```python
from build123d import *

# Parameters (mm, degrees)
BOSS_EXTRUDE1_DEPTH  = 19.05
M5_CLEARANCE_HOLE1_D = 5.5
CUT_EXTRUDE1_REACH   = 3.519
SKETCH5_W            = 20.32
SKETCH5_H            = 40.64
CUT_EXTRUDE2_REACH   = 3.519
SKETCH6_R            = 2.032


with BuildPart() as part:
    # Sketch1 → Boss-Extrude1 (new body, symmetric)
    with BuildSketch(Plane(origin=(0, 0, 0), x_dir=(0, 0, -1), z_dir=(1, 0, 0))):
        Polygon((0, 0), (28.380612245, 0), (28.380612245, 63.5), (26.861692245, 63.5), (26.861692245, 1.51892), (0, 1.51892), align=None)
    extrude(amount=BOSS_EXTRUDE1_DEPTH, both=True)

    # M5 Clearance Hole1 (through all)
    with Locations(Plane(origin=(0, 1.51892, 0), x_dir=(1, 0, 0), z_dir=(0, 1, 0))):
        with Locations((-12.7, 13.430846122), (12.7, 13.430846122)):
            Hole(M5_CLEARANCE_HOLE1_D / 2)

    # Sketch5 → Cut-Extrude1 (cut, up to next)
    with BuildSketch(Plane.XY.offset(-26.861692245), mode=Mode.PRIVATE) as cut_extrude1_sk1:
        with Locations((0, 32.50946)):
            Rectangle(SKETCH5_W, SKETCH5_H)
    cut_extrude1_tool1 = extrude(cut_extrude1_sk1.sketch, amount=-CUT_EXTRUDE1_REACH, mode=Mode.PRIVATE) & part.part
    add(cut_extrude1_tool1.solids().sort_by_distance((0, 32.50946, -26.861692))[0], mode=Mode.SUBTRACT)

    # Sketch6 → Cut-Extrude2 (cut, up to next)
    with BuildSketch(Plane.XY.offset(-26.861692245), mode=Mode.PRIVATE) as cut_extrude2_sk1:
        with Locations((-5.969, 57.50946)):
            Circle(SKETCH6_R)
    cut_extrude2_tool1 = extrude(cut_extrude2_sk1.sketch, amount=-CUT_EXTRUDE2_REACH, mode=Mode.PRIVATE) & part.part
    add(cut_extrude2_tool1.solids().sort_by_distance((-5.969, 57.50946, -26.861692))[0], mode=Mode.SUBTRACT)
    # Sketch6 → Cut-Extrude2 (cut, up to next)
    with BuildSketch(Plane.XY.offset(-26.861692245), mode=Mode.PRIVATE) as cut_extrude2_sk2:
        with Locations((5.969, 57.50946)):
            Circle(SKETCH6_R)
    cut_extrude2_tool2 = extrude(cut_extrude2_sk2.sketch, amount=-CUT_EXTRUDE2_REACH, mode=Mode.PRIVATE) & part.part
    add(cut_extrude2_tool2.solids().sort_by_distance((5.969, 57.50946, -26.861692))[0], mode=Mode.SUBTRACT)
    # Sketch6 → Cut-Extrude2 (cut, up to next)
    with BuildSketch(Plane.XY.offset(-26.861692245), mode=Mode.PRIVATE) as cut_extrude2_sk3:
        with Locations((-5.969, 7.50946)):
            Circle(SKETCH6_R)
    cut_extrude2_tool3 = extrude(cut_extrude2_sk3.sketch, amount=-CUT_EXTRUDE2_REACH, mode=Mode.PRIVATE) & part.part
    add(cut_extrude2_tool3.solids().sort_by_distance((-5.969, 7.50946, -26.861692))[0], mode=Mode.SUBTRACT)
    # Sketch6 → Cut-Extrude2 (cut, up to next)
    with BuildSketch(Plane.XY.offset(-26.861692245), mode=Mode.PRIVATE) as cut_extrude2_sk4:
        with Locations((5.969, 7.50946)):
            Circle(SKETCH6_R)
    cut_extrude2_tool4 = extrude(cut_extrude2_sk4.sketch, amount=-CUT_EXTRUDE2_REACH, mode=Mode.PRIVATE) & part.part
    add(cut_extrude2_tool4.solids().sort_by_distance((5.969, 7.50946, -26.861692))[0], mode=Mode.SUBTRACT)


solid = part.part
```
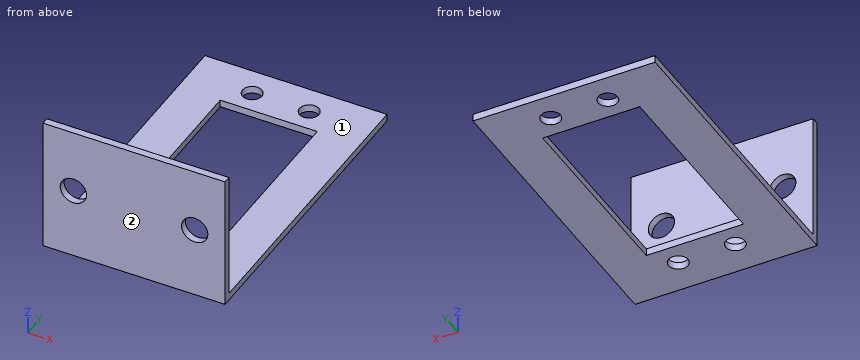
CAD build for the part. Positions are in the model's coordinates, mm. Face numbers are marked on the shaded views. A direction names the side the tool comes from. Give positions to 0.01 mm unless a question says otherwise; leave off trailing zeros. Order: outer loops, then holes, each group sorted by start corner. A loop starts at its lowest first (then second) coordinate and runs counter-clockwise, first axis right, second up.
(1) Tool access for the marked faces 1 and 2: list every direction of +Z, -Z, +X, -X, +Y, -Y with a clear straight run to the whole face (end or side of a thin tool).
(2) Drill centre lines: L1, parallel to Z at x = -12.7, y = 0.35; L2, parallel to Y at x = -3, z = -26.25; L3, parallel to Z at x = -17, y = 45. Where is each one in solid material? Low to high.
(3) Saw through at C-C, the plane x = 1. Give the cut face in (y, z), then the cut area to 3 significant figures.
(4) Saw through at B-B, the plane y = 44.5. Give the cut face in (x, z).
(5) Saw through at A-A, the plane x = -12.7. Give the cut face in (y, z), then the cut area to 3 significant figures.
(6) Flat gauge pins, fed straight in: pin 1 (5.5 mm diameter, centred on x = 5.97, y = 7.51, fed in from +Z); pin 2 (1.5 mm diameter, centred on x = 11, z = -9.5, fed in from +Y). Where does each tip first touch, or does it go through?
(7) Saw through at D-D, the plane x = -7. Give the cut face in (y, z).
Results found:
1. face 1: +Z, +X, -X, +Y
1. face 2: +Z, -Z, +X, -X, -Y
2. L1: z = -28.38 to -16.18, -10.68 to 0
2. L2: y = 0 to 1.52
2. L3: z = -28.38 to -26.86
3. outline: (0, -28.38) - (12.19, -28.38) - (12.19, -26.86) - (1.52, -26.86) - (1.52, 0) - (0, 0) - close; (52.83, -28.38) - (63.5, -28.38) - (63.5, -26.86) - (52.83, -26.86) - close
3. area: 75.5 mm2
4. outline: (-19.05, -28.38) - (-10.16, -28.38) - (-10.16, -26.86) - (-19.05, -26.86) - close; (10.16, -28.38) - (19.05, -28.38) - (19.05, -26.86) - (10.16, -26.86) - close
5. outline: (0, -28.38) - (63.5, -28.38) - (63.5, -26.86) - (1.52, -26.86) - (1.52, -16.18) - (0, -16.18) - close; (0, -10.68) - (1.52, -10.68) - (1.52, 0) - (0, 0) - close
5. area: 129 mm2
6. pin 1: stops at z = -26.86
6. pin 2: stops at y = 1.52
7. outline: (0, -28.38) - (5.76, -28.38) - (5.76, -26.86) - (1.52, -26.86) - (1.52, 0) - (0, 0) - close; (9.26, -28.38) - (12.19, -28.38) - (12.19, -26.86) - (9.26, -26.86) - close; (52.83, -28.38) - (55.76, -28.38) - (55.76, -26.86) - (52.83, -26.86) - close; (59.26, -28.38) - (63.5, -28.38) - (63.5, -26.86) - (59.26, -26.86) - close
